from build123d import *

# Parameters (mm, degrees)
F1_DEPTH = 25.4
F2_DEPTH = 6.35
F4_DEPTH = 3.175
F5_R     = 24.9785036256
F6_DEPTH = 89.916


with BuildPart() as f1:
    # F0 (on Top) → F1 (new body)
    with BuildSketch(Plane.XY):
        with BuildLine():
            Line((51.2434020638, 37.2763350606), (50.6863420601, 37.2763350606))
            ThreePointArc((50.6863420601, 37.2763350606), (13.6874964232, 0), (50.6863420601, -37.2763350606))
            Line((50.6863420601, -37.2763350606), (51.2434020638, -37.2763350606))
            Line((51.2434020638, -37.2763350606), (51.2434020638, 37.2763350606))
        make_face()
        with BuildLine():
            ThreePointArc((88.2422477007, 0), (77.4222491241, 26.2604252346), (51.2434020638, 37.2763350606))
            Line((51.2434020638, 37.2763350606), (51.2434020638, -37.2763350606))
            ThreePointArc((51.2434020638, -37.2763350606), (77.4222491241, -26.2604252346), (88.2422477007, 0))
        make_face()
    extrude(amount=F1_DEPTH)

    # F0 (on Top) → F2 (join)
    with BuildSketch(Plane.XY):
        with BuildLine():
            Line((50.6863420601, 37.2763350606), (-51.2434020638, 37.2763350606))
            Line((-51.2434020638, 37.2763350606), (-51.2434020638, -37.2763350606))
            Line((-51.2434020638, -37.2763350606), (50.6863420601, -37.2763350606))
            ThreePointArc((50.6863420601, -37.2763350606), (13.6874964232, 0), (50.6863420601, 37.2763350606))
        make_face()
    extrude(amount=F2_DEPTH)

    # F3 (on Front) → F4 (join, symmetric)
    with BuildSketch(Plane.XZ):
        Polygon((13.5906888172, 25.4415851086), (0, 0), (13.5906888172, 0), align=None)
    extrude(amount=F4_DEPTH, both=True)

    # F5 (on face) → F6 (cut)
    with BuildSketch(Plane.XY.offset(25.4)):
        with Locations((50.964872062, 0)):
            Circle(F5_R)
    extrude(amount=-F6_DEPTH, mode=Mode.SUBTRACT)


solid = f1.part
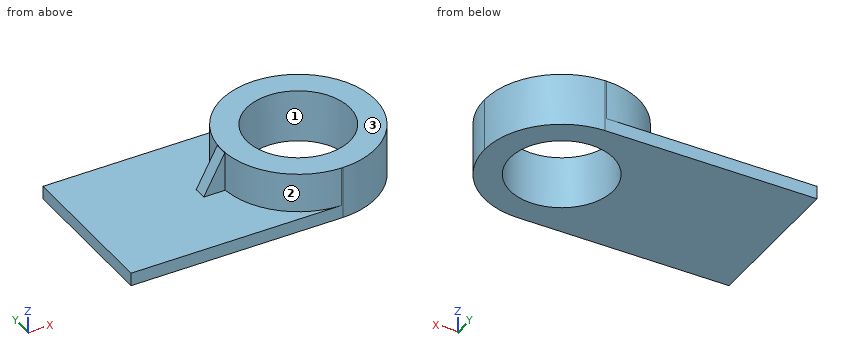
Model file for the job. Use its own axes, mm. Face numbers are marked on the shaded views. Give positions to 0.01 mm unless a question says otherwise; leave off trailing zeros. Loops run counter-clockwise (first coordinate to the right, second up) from the corner with the lowest first, then second, coordinate; pieces in that order, holes last.
Item 1: Drop flat-ended pins along their axis: P1, Ø4, axis at y = 11.5, z = 20.5, coming from the +X side; P2, Ø3, axis at x = 69, z = 13, coming from the +Y side; P3, Ø6, axis at x = 16, y = -19.5, coming from the +Z side. Give the stop position or say it passes through.
Check values:
P1: stops at x = 87.01
P2: stops at y = 33.41
P3: stops at z = 25.4
Item 2: Slice it at D-D (y = -21). Write the cut outline in (x, z).
Check values:
outline: (-51.24, 0) - (37.44, 0) - (37.44, 25.4) - (20.17, 25.4) - (20.17, 6.35) - (-51.24, 6.35) - close; (64.49, 0) - (81.76, 0) - (81.76, 25.4) - (64.49, 25.4) - close
Item 3: Slice it at C-C (y = -9). Write the cut outline in (x, z).
Check values:
outline: (-51.24, 0) - (27.66, 0) - (27.66, 25.4) - (14.79, 25.4) - (14.79, 6.35) - (-51.24, 6.35) - close; (74.27, 0) - (87.14, 0) - (87.14, 25.4) - (74.27, 25.4) - close
Item 4: Slice it at B-B (x = 68.5). Write the cut outline in (y, z), plus the area to 3 significant figures.
Check values:
outline: (-32.9, 0) - (-17.79, 0) - (-17.79, 25.4) - (-32.9, 25.4) - close; (17.79, 0) - (32.9, 0) - (32.9, 25.4) - (17.79, 25.4) - close
area: 767 mm2
Item 5: Mould opens along Y. For the marked faces 1, 2 and 3 say: +Y half, -Y half, draft (parallel to the pull), parting line (faces both ways), or undercut.
Check values:
face 1: undercut
face 2: parting line
face 3: draft
Item 6: Drill centre lines: line 1 along X through (y, z) = (2.5, 16.75); line 2 along Z through (x, y) = (-32.5, 17.5); line 3 along Y through (x, z) = (49.5, 23). Where is each one in solid material? Low to high.
Check values:
line 1: x = 8.95 to 13.59, 13.77 to 26.11, 75.82 to 88.16
line 2: z = 0 to 6.35
line 3: y = -37.25 to -24.94, 24.94 to 37.25
Item 7: Slice it at A-A (z = 12.5). Write the cut outline in (x, y) (1 decimal), plus the area to 3 significant figures.
Check values:
outline: (6.7, -3.2) - (13.6, -3.2) - (13.6, 3.2) - (6.7, 3.2) - close; (50.7, -37.3) - (51.2, -37.3) arc R37.3 ccw to (51.2, 37.3) - (50.7, 37.3) arc R37.3 ccw to start; hole circle Ø50 at (51, 0)
area: 2,450 mm2
